```python
from build123d import *

# Parameters (mm, degrees)
F0_R     = 6
F1_DEPTH = 25
F2_R     = 10
F3_DEPTH = 20


with BuildPart() as f1:
    # F0 (on Front) → F1 (new body)
    with BuildSketch(Plane.XZ):
        with BuildLine():
            Line((-125, -355), (-72.5, -355))
            Line((-72.5, -355), (-72.5, -325))
            ThreePointArc((-72.5, -325), (-76.035534, -316.464466), (-67.5, -320))
            Line((-67.5, -320), (67.5, -320))
            ThreePointArc((67.5, -320), (72.5, -315), (77.5, -320))
            ThreePointArc((77.5, -320), (76.035534, -323.535534), (72.5, -325))
            Line((72.5, -325), (72.5, -355))
            Line((72.5, -355), (125, -355))
            Line((125, -355), (252.5, 0))
            Line((252.5, 0), (0, 0))
            Line((0, 0), (-252.5, 0))
            Line((-252.5, 0), (-125, -355))
        make_face()
        with Locations((-140, -100)):
            Circle(F0_R, mode=Mode.SUBTRACT)
        with Locations((140, -100)):
            Circle(F0_R, mode=Mode.SUBTRACT)
    extrude(amount=F1_DEPTH)

    # F2 (on face) → F3 (cut)
    with BuildSketch(Plane.XZ.offset(25)):
        with Locations((-140, -100)):
            Circle(F2_R)
        with Locations((140, -100)):
            Circle(F2_R)
    extrude(amount=-F3_DEPTH, mode=Mode.SUBTRACT)


solid = f1.part
```
Model file for the job. Use its own axes, mm. A direction names the side the tool comes from. Coordinates: 2 decimals unless noted, no trailing zeros. Order: outer loops, then holes, each group sorted by start corner. A loop starts at its lowest first (then second) coordinate and runs counter-clockwise, first axis right, second up. Notation, with made-up numbers: M 10,54 L 15,54 A11 ccw 15,68 Z; hole C -4.5,40 d9. An arc over 180 degrees is marked long. Answer as CSV lines item,"result".
(1) Pull direction X, two halves, no side cores. Call faces 4 (the cylindrical face through (145.38, -15.14, -91.57)), 5 (the flat face through (-189.64, -12.32, -175.02)), 6 (the cylindrical face through (-76.15, -12.32, -316.58)), 7 (the flat face through (-4, -25, -136)): +X half, -X half, draft (parallel to the pull), parting line (faces both ways), or undercut.
Geometry says:
face 4,"undercut"
face 5,"-X half"
face 6,"undercut"
face 7,"draft"
(2) 3-axis set-ups, long thin cutter, end or side, ignore diameter. For faces 1 (the flat face through (-72.5, -12, -340)), 2 (the flat face through (-4, 0, -136)), 3 (the flat face through (-133, -5, -100)): which of +Z, -Z, +X, -X, +Y, -Y reach the whole face in a straight line?
Geometry says:
face 1,"-Z, +Y, -Y"
face 2,"+Z, -Z, +X, -X, +Y"
face 3,"-Y"
(3) Band-saw the part on A-A, the plane y = -15. List the corners of the cut face in (x, z).
Geometry says:
outline,"M -252.5,0 L -125,-355 L -72.5,-355 L -72.5,-325 A5 cw long -67.5,-320 L 67.5,-320 A5 cw long 72.5,-325 L 72.5,-355 L 125,-355 L 252.5,0 Z; hole C -140,-100 d20; hole C 140,-100 d20"
(4) Band-saw the part on C-C, the plane x = -140. List the corners of the cut face in (y, z), then the cut area to 3 significant figures.
Geometry says:
outline,"M -25,-313.24 L 0,-313.24 L 0,-106 L -5,-106 L -5,-110 L -25,-110 Z; M -25,-90 L -5,-90 L -5,-94 L 0,-94 L 0,0 L -25,0 Z"
area,"7,370 mm2"
(5) Flat gauge pins, fed straight in: pin 1 (8 mm diameter, centred on y = -8.5, z = -185, fed in from -X); pin 2 (8 mm diameter, centred on y = -13.5, z = -84.5, fed in from +X); pin 3 (6 mm diameter, centred on x = -143.5, z = -98.5, fed in from -Y); pin 4 (5 mm diameter, centred on x = 2, z = -217, fed in from +Y). Where does each tip first touch, or does it go through?
Geometry says:
pin 1,"stops at x = -187.49"
pin 2,"stops at x = 223.59"
pin 3,"stops at y = -5"
pin 4,"stops at y = 0"
(6) Band-saw the part on B-B, the plane z = -100. List the corners of the cut face in (x, y), then the cut area to 3 significant figures.
Geometry says:
outline,"M -216.58,-25 L -150,-25 L -150,-5 L -146,-5 L -146,0 L -216.58,0 Z; M -134,-5 L -130,-5 L -130,-25 L 130,-25 L 130,-5 L 134,-5 L 134,0 L -134,0 Z; M 146,-5 L 150,-5 L 150,-25 L 216.58,-25 L 216.58,0 L 146,0 Z"
area,"9,910 mm2"
(7) Band-saw the part on D-D, the plane z = -181. List the corners of the cut face in (x, y).
Geometry says:
outline,"M -187.49,-25 L 187.49,-25 L 187.49,0 L -187.49,0 Z"
(8) Wall check: line 1 along X through (y, z) = (-13.25, -108.5); line 2 along X through (y, z) = (-1.65, -100); line 3 along X through (y, z) = (-22, -65). Give the ranges that are in metal, low to high.
Geometry says:
line 1,"x = -213.53 to -145.27, -134.73 to 134.73, 145.27 to 213.53"
line 2,"x = -216.58 to -146, -134 to 134, 146 to 216.58"
line 3,"x = -229.15 to 229.15"
